The model under review builds one solid part; all positions refer to its coordinate system, in mm. A direction names the side the tool comes from. Round coordinates to 2 decimals unless told otherwise and drop trailing zeros. Order: outer loops, then holes, each group sorted by start corner. A loop starts at its lowest first (then second) coordinate and runs counter-clockwise, first axis right, second up. Notation, with made-up numbers: (-31, -26.5) -> (-23, -26.5) arc R27 cw to (-23, 5.5) -> close; hole circle Ø11 at (-29.5, 62.25). An arc over 180 degrees is marked (long way). Use a Markdown table: item, result. Add a question column.
```python
from build123d import *

# Parameters (mm, degrees)
F0_R     = 11.1125
F1_DEPTH = 88.9
F2_R     = 6.35
F3_DEPTH = 88.9
F4_R     = 1.7907
F5_DEPTH = 22.225


with BuildPart() as f1:
    # F0 (on Top) → F1 (new body)
    with BuildSketch(Plane.XY):
        Circle(F0_R)
    extrude(amount=F1_DEPTH)

    # F2 (on face) → F3 (cut)
    with BuildSketch(Plane.XY.offset(88.9)):
        Circle(F2_R)
    extrude(amount=-F3_DEPTH, mode=Mode.SUBTRACT)

    # F4 (on Front) → F5 (cut)
    with BuildSketch(Plane.XZ):
        with Locations((0, 12.7)):
            Circle(F4_R)
        with Locations((0, 76.2)):
            Circle(F4_R)
    extrude(amount=-F5_DEPTH, mode=Mode.SUBTRACT)


solid = f1.part
```
Q1. Add section D-D (x = 4). Write out the cut boundary in (y, z), then the cut area to 3 significant figures.
Q2. Add section B-B (y = 0). Write out the cut boundary in (x, z), then the cut area to 3 significant figures.
Q3. Wall thickness on line 1 (Z direction, x = 0, y = 10); line 2 (Y direction, x = 0, z = 56); line 3 (Y direction, x = 2.5, z = 26.5): over which ranges is each line inside the solid? List them lowest first. Write a range as [from, to].
Q4. Add section A-A (x = 0). Write out the cut boundary in (y, z).
Q5. Mouldability with a two-part tool opening along Z and no side actions: class faces 1 (the flat face through (5, -5, 88.9)), 2 (the cylindrical face through (-1.38, -6.2, 45.07)), 3 (the cylindrical face through (1.654, 8.565, 75.514)) as pulls with the +Z half, pulls with the -Z half, needs draft (parallel to the pull), parting line crosses it, or undercut.
Q6. Machinability: for faces 4 (the cylindrical face through (10.6, 3.34, 43.83)), 5 (the cylindrical face through (1.654, 8.565, 12.014)), which of the approach directions +Z, -Z, +X, -X, +Y, -Y give a long, thin tool a straight path to every point of the face, cutting with its end or side? Answer none if there is none.
Q7. Insertion check: pin 1 (2 mm diameter, centred on x = -8, z = 11.5, fed in from -Y); pin 2 (7.5 mm diameter, centred on x = 0, y = 0, fed in from +Z); pin 3 (1 mm diameter, centred on y = 6.5, z = 71.5, fed in from +X); pin 4 (3 mm diameter, centred on x = -2, z = 38, fed in from +Y). Each pin has a flat end and moves straight along its axis. Give the tip position at first contact, or say it passes through.
Report:
| question | item | result |
|---|---|---|
| 1 | outline | (-10.37, 0) -> (-4.93, 0) -> (-4.93, 88.9) -> (-10.37, 88.9) -> close; (4.93, 0) -> (10.37, 0) -> (10.37, 88.9) -> (4.93, 88.9) -> close |
| 1 | area | 966 mm² |
| 2 | outline | (-11.11, 0) -> (-6.35, 0) -> (-6.35, 88.9) -> (-11.11, 88.9) -> close; (6.35, 0) -> (11.11, 0) -> (11.11, 88.9) -> (6.35, 88.9) -> close |
| 2 | area | 847 mm² |
| 3 | line 1 | z = [0, 10.91], [14.49, 74.41], [77.99, 88.9] |
| 3 | line 2 | y = [-11.11, -6.35], [6.35, 11.11] |
| 3 | line 3 | y = [-10.83, -5.84], [5.84, 10.83] |
| 4 | outline | (-11.11, 0) -> (-6.35, 0) -> (-6.35, 88.9) -> (-11.11, 88.9) -> close; (6.35, 0) -> (11.11, 0) -> (11.11, 10.91) -> (6.35, 10.91) -> close; (6.35, 14.49) -> (11.11, 14.49) -> (11.11, 74.41) -> (6.35, 74.41) -> close; (6.35, 77.99) -> (11.11, 77.99) -> (11.11, 88.9) -> (6.35, 88.9) -> close |
| 5 | face 1 | pulls with the +Z half |
| 5 | face 2 | needs draft |
| 5 | face 3 | undercut |
| 6 | face 4 | +Z, -Z |
| 6 | face 5 | +Y |
| 7 | pin 1 | stops at y = -8.63 |
| 7 | pin 2 | passes through |
| 7 | pin 3 | stops at x = 9.35 |
| 7 | pin 4 | stops at y = 11.1 |
